Build history of the part. All positions in model axes, mm. Face numbers are marked on the shaded views. A direction names the side the tool comes from. Round coordinates to 2 decimals unless told otherwise and drop trailing zeros. Write each loop counter-clockwise with the first axis right and the second up, starting at its lowest first coordinate (ties: lowest second). Pieces come first, ordered by that corner, then holes.
1) Saw through at A-A (x = 0). Write the cut outline in (y, z), plus the area to 3 significant figures.
2) Which spindle directions (+Z, -Z, +X, -X, +Y, -Y) get a long thin tool onto all of the face, cutting with end or side? Do the marked faces 1, 2 and 3. Say none if no direction does.
3) Wall check: probe 1 along Y at (x, z) = (0, -2.45); probe 2 along Z at (x, y) = (0, 4.25); probe 3 along X at (y, z) = (0, 1.9). Give the ranges that are in metal, low to high.
4) Pull direction X, two halves, no side cores. Call the marked faces 4, 5 and 6: +X half, -X half, draft (parallel to the pull), parting line (faces both ways), or undercut.
5) Saw through at D-D (y = -3.25). Write the cut outline in (x, z).
6) Flat gauge pins, fed straight in: pin 1 (1.5 mm diameter, centred on x = 5.5, y = 3, fed in from -Z); pin 2 (1.3 mm diameter, centred on x = -0.5, y = 1, fed in from +Z); pin 3 (1 mm diameter, centred on x = 7, z = 1, fed in from -Y); pin 4 (1.2 mm diameter, centred on x = 0, y = 0, fed in from -Z). Where does each tip first touch, or does it go through?
7) Saw through at C-C (z = -1.5). Write the cut outline in (x, y).
Autodesk Fusion 360 part; units mm, degrees
sketch "Horn Body" plane through (0, 0, 0) normal (0, 0, 1) x (1, 0, 0)
  circle A0 centre (0, 0) radius 10
  dimension "d1" = 20
extrude "Extrude1" add sketch "Horn Body" along normal blind 1.5
sketch "Connector" plane through (0, 0, 0) normal (0, 0, -1) x (1, 0, 0)
  circle A0 centre (0, 0) radius 10
  circle A1 centre (0, 0) radius 2.5
  circle A2 centre (0, 0) radius 3.5
  dimension "d4" = 5
  dimension "d5" = 7
extrude "Extrude2" add sketch "Connector" along normal blind 3.5 contours A2
sketch "Screw Hole" plane through (0, 0, 1.5) normal (0, 0, 1) x (-1, 0, 0)
  circle A0 centre (0, 0) radius 10
  circle A1 centre (0, 0) radius 2.75
  circle A2 centre (0, 0) radius 2.25
  circle A3 centre (0, 0) radius 1
  dimension "d8" = 5.5
  dimension "d9" = 4.5
  dimension "d10" = 2
extrude "Extrude3" add sketch "Screw Hole" along normal blind 0.5 contours A1
extrude "Extrude4" cut sketch "Screw Hole" against normal blind 1.5 contours A3
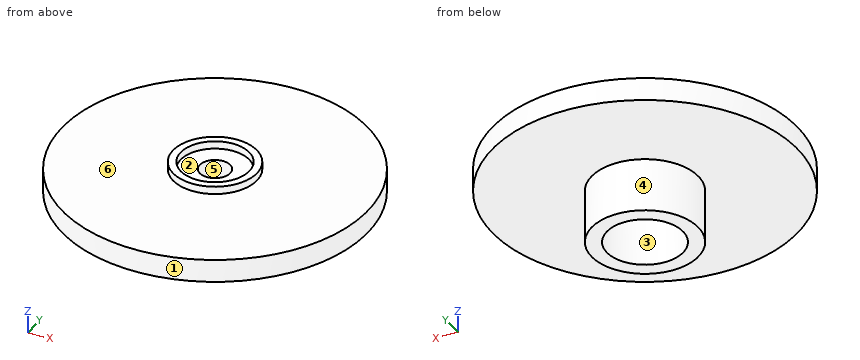
Evaluation:
1. outline: (-10, 0) - (-3.5, 0) - (-3.5, -3.5) - (-2.5, -3.5) - (-2.5, 0) - (-1, 0) - (-1, 1.5) - (-2.25, 1.5) - (-2.25, 2) - (-2.75, 2) - (-2.75, 1.5) - (-10, 1.5) - close; (1, 0) - (2.5, 0) - (2.5, -3.5) - (3.5, -3.5) - (3.5, 0) - (10, 0) - (10, 1.5) - (2.75, 1.5) - (2.75, 2) - (2.25, 2) - (2.25, 1.5) - (1, 1.5) - close
1. area: 34.5 mm2
2. face 1: +Z, -Z
2. face 2: +Z
2. face 3: -Z
3. probe 1: y = -3.5 to -2.5, 2.5 to 3.5
3. probe 2: z = 0 to 1.5
3. probe 3: x = -2.75 to -2.25, 2.25 to 2.75
4. face 4: parting line
4. face 5: undercut
4. face 6: draft
5. outline: (-9.46, 0) - (-1.3, 0) - (-1.3, -3.5) - (1.3, -3.5) - (1.3, 0) - (9.46, 0) - (9.46, 1.5) - (-9.46, 1.5) - close
6. pin 1: stops at z = 0
6. pin 2: stops at z = 1.5
6. pin 3: stops at y = -7.6
6. pin 4: passes through
7. outline: circle Ø7 at (0, 0); hole circle Ø5 at (0, 0)
